The listing builds one solid part. Answer for the finished solid, in the listing's coordinates (mm). A direction names the side the tool comes from. Round coordinates to 2 decimals unless told otherwise and drop trailing zeros. Order: outer loops, then holes, each group sorted by start corner. A loop starts at its lowest first (then second) coordinate and runs counter-clockwise, first axis right, second up. Notation, with made-up numbers: (-39, 23.5) -> (-31, 23.5) arc R23 cw to (-31, 42.5) -> close; hole circle Ø8 at (-7, 69.5). An arc over 180 degrees is marked (long way). Answer in a Markdown table with one row per item. Add a question column.
```python
from build123d import *

# Parameters (mm, degrees)
SKETCH1_W           = 199
SKETCH1_H           = 153
BOSS_EXTRUDE1_DEPTH = 5
SKETCH2_W           = 153
SKETCH2_H           = 199
SKETCH2_W_2         = 82
SKETCH2_H_2         = 122
SKETCH2_H_3         = 62
SKETCH2_W_3         = 56
SKETCH2_H_4         = 189
BOSS_EXTRUDE2_DEPTH = 10
SKETCH3_W           = 153
SKETCH3_H           = 199
SKETCH3_W_2         = 143
SKETCH3_H_2         = 189
BOSS_EXTRUDE3_DEPTH = 20
SKETCH4_W           = 6
SKETCH4_H           = 6
BOSS_EXTRUDE4_DEPTH = 3
FILLET1_R           = 6
SKETCH5_W           = 70
SKETCH5_H           = 5
CUT_EXTRUDE1_DEPTH  = 27
SKETCH6_R           = 1.75
CUT_EXTRUDE2_DEPTH  = 5


with BuildPart() as part:
    # Sketch1 → Boss-Extrude1 (new body)
    with BuildSketch(Plane(origin=(0, 0, 0), x_dir=(0, 1, 0), z_dir=(0, 0, 1))):
        with Locations((99.5, 76.5)):
            Rectangle(SKETCH1_W, SKETCH1_H)
    extrude(amount=-BOSS_EXTRUDE1_DEPTH)

    # Sketch2 → Boss-Extrude2 (add)
    with BuildSketch(Plane.XY):
        with Locations((-76.5, 99.5)):
            Rectangle(SKETCH2_W, SKETCH2_H)
        with Locations((-46, 66)):
            Rectangle(SKETCH2_W_2, SKETCH2_H_2, mode=Mode.SUBTRACT)
        with Locations((-46, 163)):
            Rectangle(SKETCH2_W_2, SKETCH2_H_3, mode=Mode.SUBTRACT)
        with Locations((-120, 99.5)):
            Rectangle(SKETCH2_W_3, SKETCH2_H_4, mode=Mode.SUBTRACT)
    extrude(amount=BOSS_EXTRUDE2_DEPTH)

    # Sketch3 → Boss-Extrude3 (add)
    with BuildSketch(Plane.XY.offset(10)):
        with Locations((-76.5, 99.5)):
            Rectangle(SKETCH3_W, SKETCH3_H)
        with Locations((-76.5, 99.5)):
            Rectangle(SKETCH3_W_2, SKETCH3_H_2, mode=Mode.SUBTRACT)
    extrude(amount=BOSS_EXTRUDE3_DEPTH)

    # Sketch4 → Boss-Extrude4 (add)
    with BuildSketch(Plane.XY):
        with Locations((-84, 124)):
            Rectangle(SKETCH4_W, SKETCH4_H)
        with Locations((-8, 124)):
            Rectangle(SKETCH4_W, SKETCH4_H)
        with Locations((-8, 8)):
            Rectangle(SKETCH4_W, SKETCH4_H)
        with Locations((-84, 8)):
            Rectangle(SKETCH4_W, SKETCH4_H)
    extrude(amount=BOSS_EXTRUDE4_DEPTH)

    # Fillet1
    fillet1_edges = [part.edges().sort_by_distance(p)[0] for p in [
        (-81, 11, 1.5),
        (-11, 11, 1.5),
        (-81, 121, 1.5),
        (-11, 121, 1.5),
    ]]
    fillet(fillet1_edges, radius=FILLET1_R - 0.0001)  # a hair under: the kernel refuses the full size

    # Sketch5 → Cut-Extrude1 (cut)
    with BuildSketch(Plane.XY.offset(30)):
        with Locations((-46, 2.5)):
            Rectangle(SKETCH5_W, SKETCH5_H)
    extrude(amount=-CUT_EXTRUDE1_DEPTH, mode=Mode.SUBTRACT)

    # Sketch6 → Cut-Extrude2 (cut)
    with BuildSketch(Plane(origin=(-5, 0, 0), x_dir=(0, -1, 0), z_dir=(-1, 0, 0))):
        with Locations((-179, 24.75)):
            Circle(SKETCH6_R)
    extrude(amount=-CUT_EXTRUDE2_DEPTH, mode=Mode.SUBTRACT)


solid = part.part
```
1. The mould has two halves that part along X. Classify faces 1 (the flat face through (-151, 115, 30)), 2 (the flat face through (-47, 65, 0)): released by +X, released by -X, zero draft, split by the parting line, or undercut.
2. For faces 3 (the flat face through (-11, 2, 17)), 4 (the flat face through (-87, 163, 5)), determine the directions among +Z, -Z, +X, -X, +Y, -Y from which every point of the face is accessible in a straight line to the end or side of a thin tool.
3. Each of these flat-tipped pins is pushed along its axis until it touches: pin 1 (1.8 mm diameter, centred on x = -8, y = 124.5, fed in from +Z); pin 2 (4 mm diameter, centred on x = -56, y = 174.5, fed in from +Z). Where does it stop, or does it pass through?
4. The part is cut by section B-B (x = -128.5). Give the vertices of the cut face in (y, z), then the cut area to 4 significant figures.
5. The part is cut by section C-C (z = 13). Give the vertices of the cut face in (x, y), then the cut area to 3 significant figures.
6. Straight lines are drawn through the part: line 1 along X through (y, z) = (59, 12.5); line 2 along X through (y, z) = (36.5, 4); line 3 along Y through (x, z) = (-107.5, 16.5). For each, find the intervals that lie inside material, in ascending order.
7. The part is cut by section A-A (y = 172.5). Give the vertices of the cut face in (x, z), then the cut area to 4 significant figures.
8. The part is cut by section D-D (y = 124). Give the vertices of the cut face in (x, z).
Report:
| question | item | result |
|---|---|---|
| 1 | face 1 | zero draft |
| 1 | face 2 | undercut |
| 2 | face 3 | +Z, -Y |
| 2 | face 4 | +Z |
| 3 | pin 1 | stops at z = 3 |
| 3 | pin 2 | stops at z = 0 |
| 4 | outline | (0, -5) -> (199, -5) -> (199, 30) -> (194, 30) -> (194, 0) -> (5, 0) -> (5, 30) -> (0, 30) -> close |
| 4 | area | 1,295 mm^2 |
| 5 | outline | (-153, 0) -> (-81, 0) -> (-81, 5) -> (-148, 5) -> (-148, 194) -> (-5, 194) -> (-5, 5) -> (-11, 5) -> (-11, 0) -> (0, 0) -> (0, 199) -> (-153, 199) -> close |
| 5 | area | 3,070 mm^2 |
| 6 | line 1 | x = -153 to -148, -5 to 0 |
| 6 | line 2 | x = -153 to -148, -92 to -87, -5 to 0 |
| 6 | line 3 | y = 0 to 5, 194 to 199 |
| 7 | outline | (-153, -5) -> (0, -5) -> (0, 30) -> (-5, 30) -> (-5, 0) -> (-87, 0) -> (-87, 10) -> (-92, 10) -> (-92, 0) -> (-148, 0) -> (-148, 30) -> (-153, 30) -> close |
| 7 | area | 1,115 mm^2 |
| 8 | outline | (-153, -5) -> (0, -5) -> (0, 30) -> (-5, 30) -> (-5, 3) -> (-10.2, 3) -> (-10.2, 0) -> (-81.8, 0) -> (-81.8, 3) -> (-87, 3) -> (-87, 10) -> (-92, 10) -> (-92, 0) -> (-148, 0) -> (-148, 30) -> (-153, 30) -> close |
